Can you work these out from the model? Positions are in its coordinate system, mm. A direction names the side the tool comes from. Give positions to 0.01 mm unless a question says otherwise; leave off trailing zeros. Order: outer loops, then holes, each group sorted by start corner. A loop starts at its lowest first (then second) coordinate and runs counter-clockwise, first axis right, second up. Notation, with made-up numbers: M 74.25,56 L 117.25,56 A32 ccw 117.25,84 Z; hole C 41.25,1 d4. An arc over 180 degrees is marked long. Write each question's results on one line, items separated by ' | '.
from build123d import *

# Parameters (mm, degrees)
SKETCH1_W                 = 33
SKETCH1_H                 = 33
SKETCH1_R                 = 7.5
BOSS_EXTRUDE1_DEPTH       = 5
F_2_56_TAPPED_HOLE4_D     = 1.778
F_2_56_TAPPED_HOLE4_DEPTH = 7.46583491
F_2_56_TAPPED_HOLE4_TIP   = 0.53416509
F_2_56_TAPPED_HOLE5_D     = 1.778
F_2_56_TAPPED_HOLE5_DEPTH = 7.46583491
F_2_56_TAPPED_HOLE5_TIP   = 0.53416509
F_2_56_TAPPED_HOLE6_D     = 1.778
F_2_56_TAPPED_HOLE6_DEPTH = 7.46583491
F_2_56_TAPPED_HOLE6_TIP   = 0.53416509
F_2_56_TAPPED_HOLE7_D     = 1.778
F_2_56_TAPPED_HOLE7_DEPTH = 7.46583491
F_2_56_TAPPED_HOLE7_TIP   = 0.53416509


with BuildPart() as part:
    # Sketch1 → Boss-Extrude1 (new body)
    with BuildSketch(Plane(origin=(0, 0, 0), x_dir=(1, 0, 0), z_dir=(0, 1, 0))):
        Rectangle(SKETCH1_W, SKETCH1_H)
        Circle(SKETCH1_R, mode=Mode.SUBTRACT)
    extrude(amount=BOSS_EXTRUDE1_DEPTH)

    # #2-56 Tapped Hole4
    with Locations(Plane.XY.offset(16.5)):
        with Locations((0, 2.5)):
            Hole(F_2_56_TAPPED_HOLE4_D / 2, depth=F_2_56_TAPPED_HOLE4_DEPTH)
            with Locations((0, 0, -(F_2_56_TAPPED_HOLE4_DEPTH + F_2_56_TAPPED_HOLE4_TIP / 2))):  # 118° drill point
                Cone(0, F_2_56_TAPPED_HOLE4_D / 2, F_2_56_TAPPED_HOLE4_TIP, mode=Mode.SUBTRACT)

    # #2-56 Tapped Hole5
    with Locations(Plane(origin=(0, 0, -16.5), x_dir=(-1, 0, 0), z_dir=(0, 0, -1))):
        with Locations((0, 2.5)):
            Hole(F_2_56_TAPPED_HOLE5_D / 2, depth=F_2_56_TAPPED_HOLE5_DEPTH)
            with Locations((0, 0, -(F_2_56_TAPPED_HOLE5_DEPTH + F_2_56_TAPPED_HOLE5_TIP / 2))):  # 118° drill point
                Cone(0, F_2_56_TAPPED_HOLE5_D / 2, F_2_56_TAPPED_HOLE5_TIP, mode=Mode.SUBTRACT)

    # #2-56 Tapped Hole6
    with Locations(Plane(origin=(16.5, 0, 0), x_dir=(0, 0, -1), z_dir=(1, 0, 0))):
        with Locations((0, 2.5)):
            Hole(F_2_56_TAPPED_HOLE6_D / 2, depth=F_2_56_TAPPED_HOLE6_DEPTH)
            with Locations((0, 0, -(F_2_56_TAPPED_HOLE6_DEPTH + F_2_56_TAPPED_HOLE6_TIP / 2))):  # 118° drill point
                Cone(0, F_2_56_TAPPED_HOLE6_D / 2, F_2_56_TAPPED_HOLE6_TIP, mode=Mode.SUBTRACT)

    # #2-56 Tapped Hole7
    with Locations(Plane.ZY.offset(16.5)):
        with Locations((0, 2.5)):
            Hole(F_2_56_TAPPED_HOLE7_D / 2, depth=F_2_56_TAPPED_HOLE7_DEPTH)
            with Locations((0, 0, -(F_2_56_TAPPED_HOLE7_DEPTH + F_2_56_TAPPED_HOLE7_TIP / 2))):  # 118° drill point
                Cone(0, F_2_56_TAPPED_HOLE7_D / 2, F_2_56_TAPPED_HOLE7_TIP, mode=Mode.SUBTRACT)


solid = part.part
(1) Imagine slicing it at D-D, the plane x = 4. Write out the boundary of the cut face in (y, z), plus the area to 3 significant figures.
Data:
outline: M 0,-16.5 L 5,-16.5 L 5,-6.34 L 0,-6.34 Z; M 0,6.34 L 5,6.34 L 5,16.5 L 0,16.5 Z | area: 102 mm2
(2) We'd pull the mould along Y, two halves only. Please class faces 1 (the face through (0, 5, -8)), 2 (the face through (-7.493, 2.465, -0.33)), 3 (the face through (12.71, 3.38, -0.12)): +Y half, -Y half, draft (parallel to the pull), parting line (faces both ways), or undercut.
Data:
face 1: +Y half | face 2: draft | face 3: undercut
(3) Imagine slicing it at C-C, the plane x = -10. Write out the boundary of the cut face in (y, z), plus the area to 3 significant figures.
Data:
outline: M 0,-16.5 L 5,-16.5 L 5,16.5 L 0,16.5 Z; hole C 2.5,0 d1.78 | area: 163 mm2
(4) Imagine slicing it at B-B, the plane y = 0.85. Write out the boundary of the cut face in (x, z).
Data:
outline: M -16.5,-16.5 L 16.5,-16.5 L 16.5,16.5 L -16.5,16.5 Z; hole C 0,0 d15
(5) Imagine slicing it at A-A, the plane z = -4.5. Write out the boundary of the cut face in (x, y).
Data:
outline: M -16.5,0 L -6,0 L -6,5 L -16.5,5 Z; M 6,0 L 16.5,0 L 16.5,5 L 6,5 Z
(6) I need wall thicknesses on L1, parallel to Z at x = -11, y = 2.5; L2, parallel to Y at x = 11, z = 0. Which ranges of each line are inside material? Lowest first, please. Write a range as from..to.
Data:
L1: z = -16.5..-0.89, 0.89..16.5 | L2: y = 0..1.61, 3.39..5
(7) For faces 4 (the face through (0, 1, 16.5)), 5 (the face through (-0.12, 3.38, -12.71)), 6 (the face through (0.12, 3.38, 12.71)), 7 (the face through (-12.71, 3.38, 0.12)), which set-ups out of +Z, -Z, +X, -X, +Y, -Y let a thin tool reach every point of the face, with its end or its side?
Data:
face 4: +Z, +X, -X, +Y, -Y | face 5: -Z | face 6: +Z | face 7: -X
(8) Will this pin go through, and if not, where does the flat tip stop? P1, Ø1.1, axis at x = 0, y = 2.5, coming from the -Z side.
Data:
P1: stops at z = -8.83
